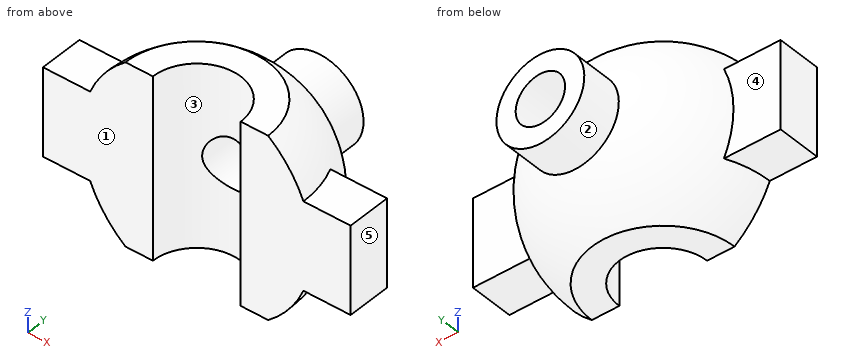
```python
from build123d import *

# Parameters (mm, degrees)
REVOLVE_2_ANGLE         = 180
EXTRUDE_1_REACH         = 59.297
EXTRUDE_1_END_RADIUS    = 21
SKETCH_3_W              = 16
SKETCH_3_H              = 8
EXTRUDE_2_REACH         = 46.204
EXTRUDE_2_END_RADIUS    = 21
SKETCH_6_R              = 8
SKETCH_7_R              = 4.5
CUT_EXTRUDE_1_DEPTH     = 45.204072223
SKETCH_8_R              = 8
CUT_EXTRUDE_2_DEPTH     = 2500
CUT_EXTRUDE_START       = -27
CUT_EXTRUDE_3_OUTLINE_W = 28
CUT_EXTRUDE_3_OUTLINE_H = 4.5
CUT_EXTRUDE_3_DEPTH     = 12.990381057


# Read off the part's stored shape, not the designer's step: 切除-拉伸3
with BuildPart() as part:
    # 草图2 → 旋转2 (revolve)
    with BuildSketch(Plane(origin=(0, 0, 0), x_dir=(1, 0, 0), z_dir=(0, 1, 0))):
        with BuildLine():
            Line((-2.539892785, -20.845837586), (2.539892785, 20.845837586))
            ThreePointArc((2.539892785, 20.845837586), (-20.845837586, 2.539892785), (-2.539892785, -20.845837586))
        make_face()
    revolve(axis=Axis((-2.539892785, 0, 20.845837586), (0.12094727545633621, 0, -0.9926589326448885)), revolution_arc=REVOLVE_2_ANGLE)

    # 凸台-拉伸1: up to this sphere (the profile starts outside it)
    extrude_1_end = Location((0, 0, 0)) * Sphere(EXTRUDE_1_END_RADIUS, mode=Mode.PRIVATE)
    # 草图3 → 凸台-拉伸1 (add, up to the surface)
    with BuildSketch(Plane(origin=(28, 0, 0), x_dir=(0, 0, -1), z_dir=(1, 0, 0)), mode=Mode.PRIVATE) as extrude_1_sk1:
        with Locations((0, 4)):
            Rectangle(SKETCH_3_W, SKETCH_3_H)
    extrude_1_tool1 = extrude(extrude_1_sk1.sketch, amount=-EXTRUDE_1_REACH, mode=Mode.PRIVATE) - extrude_1_end
    extrude_1 = extrude_1_tool1.solids().sort_by_distance((28, 4, 0))[0]
    add(extrude_1)

    # 镜向1: 凸台-拉伸1 across plane
    add(extrude_1.mirror(Plane(origin=(0, 0, 0), x_dir=(0, 0, 1), z_dir=(1, 0, 0))))

    # 凸台-拉伸2: up to this sphere (the profile starts outside it)
    extrude_2_end = Location((0, 0, 0)) * Sphere(EXTRUDE_2_END_RADIUS, mode=Mode.PRIVATE)
    # 草图6 → 凸台-拉伸2 (add, up to the surface)
    with BuildSketch(Plane(origin=(0, 27, 0), x_dir=(1, 0, 0), z_dir=(0, 1, 0)), mode=Mode.PRIVATE) as extrude_2_sk1:
        with Locations(Location((0, 0, 0), (0, 0, 270))):
            Circle(SKETCH_6_R)
    extrude_2_tool1 = extrude(extrude_2_sk1.sketch, amount=-EXTRUDE_2_REACH, mode=Mode.PRIVATE) - extrude_2_end
    add(extrude_2_tool1.solids().sort_by_distance((0, 27, 0))[0])

    # 草图7 → 切除-拉伸1 (cut, through all)
    with BuildSketch(Plane(origin=(0, 27, 0), x_dir=(1, 0, 0), z_dir=(0, 1, 0))):
        with Locations(Location((0, 0, 0), (0, 0, 270))):
            Circle(SKETCH_7_R)
    extrude(amount=-CUT_EXTRUDE_1_DEPTH, mode=Mode.SUBTRACT)

    # 草图8 → 切除-拉伸2 (cut, symmetric)
    with BuildSketch(Plane.XY):
        Circle(SKETCH_8_R)
    extrude(amount=CUT_EXTRUDE_2_DEPTH, both=True, mode=Mode.SUBTRACT)

    # 切除-拉伸3 outline → 切除-拉伸3 (cut)
    with BuildSketch(Plane(origin=(0, 27, 0), x_dir=(1, 0, 0), z_dir=(0, 1, 0)).offset(CUT_EXTRUDE_START)):
        with Locations((0, 18.75)):
            Rectangle(CUT_EXTRUDE_3_OUTLINE_W, CUT_EXTRUDE_3_OUTLINE_H)
        with Locations((0, -18.75)):
            Rectangle(CUT_EXTRUDE_3_OUTLINE_W, CUT_EXTRUDE_3_OUTLINE_H)
    extrude(amount=CUT_EXTRUDE_3_DEPTH, mode=Mode.SUBTRACT)


solid = part.part
```
Read the model definition and answer for the solid it produces. Units are mm, in the model's axes. Face numbers are marked on the shaded views. A direction names the side the tool comes from. Give positions to 0.01 mm unless a question says otherwise; leave off trailing zeros. Loops run counter-clockwise (first coordinate to the right, second up) from the corner with the lowest first, then second, coordinate; pieces in that order, holes last.
Item 1: For the marked faces 1 and 2, determine the directions among +Z, -Z, +X, -X, +Y, -Y from which every point of the face is accessible in a straight line to the end or side of a thin tool.
Item 2: Find the intervals of material crossed by line 1 along X through (y, z) = (21.5, 0); line 2 along X through (y, z) = (18.75, 0); line 3 along Z through (x, y) = (-1.5, 15), in increasing order.
Item 3: The part is cut by section B-B (y = 5.75). Write down the section's boundary in (x, z).
Item 4: Each of these flat-tipped pins is pushed along its axis until it touches: pin 1 Ø11.5 at (x, z) = (21, 3.5) entering from +Y; pin 2 Ø6.5 at (x, y) = (22.5, 4.5) entering from +Z; pin 3 Ø5 at (x, z) = (-22.5, 1) entering from +Y; pin 4 Ø6 at (x, z) = (-5, 8.5) entering from +Y. Where does it stop, or does it pass through?
Item 5: The mould has two halves that part along X. Classify the marked faces 3, 4 and 5: released by +X, released by -X, zero draft, split by the parting line, or undercut.
Item 6: The part is cut by section A-A (z = 0). Write down the section's boundary in (x, y), and give its area (3 significant figures).
Item 7: The part is cut by section D-D (x = 21.5). Write down the section's boundary in (y, z), and give its area (3 significant figures).
Item 8: The part is cut by section C-C (y = 25.25). Write down the section's boundary in (x, z).
Taken from the geometry:
1. face 1: +Z, -Z, +X, -X, -Y
1. face 2: +Y
2. line 1: x = -8 to -4.5, 4.5 to 8
2. line 2: x = -9.46 to -4.5, 4.5 to 9.46
2. line 3: z = -14.62 to -4.24, 4.24 to 14.62
3. outline: (-28, -8) - (-18.55, -8) arc R20.2 ccw to (-11.65, -16.5) - (-5.56, -16.5) - (-5.56, 16.5) - (-11.65, 16.5) arc R20.2 ccw to (-18.55, 8) - (-28, 8) - close; (5.56, -16.5) - (11.65, -16.5) arc R20.2 ccw to (18.55, -8) - (28, -8) - (28, 8) - (18.55, 8) arc R20.2 ccw to (11.65, 16.5) - (5.56, 16.5) - close
4. pin 1: stops at y = 14.13
4. pin 2: stops at z = 8
4. pin 3: stops at y = 8
4. pin 4: stops at y = 27
5. face 3: undercut
5. face 4: zero draft
5. face 5: released by +X
6. outline: (-28, 0) - (-8, 0) arc R8 cw to (-4.5, 6.61) - (-4.5, 27) - (-8, 27) - (-8, 19.42) arc R21 ccw to (-19.42, 8) - (-28, 8) - close; (4.5, 6.61) arc R8 cw to (8, 0) - (28, 0) - (28, 8) - (19.42, 8) arc R21 ccw to (8, 19.42) - (8, 27) - (4.5, 27) - close
6. area: 642 mm2
7. outline: (0, -8) - (8, -8) - (8, 8) - (0, 8) - close
7. area: 128 mm2
8. outline: circle Ø16 at (0, 0); hole circle Ø9 at (0, 0)
